The drawing under review shows one solid part. Ordinate dimensions are in mm from its lowest x, y, z. A direction names the side the tool comes from. Give positions to 0.01 mm unless a question says otherwise; leave off trailing zeros. Write each loop counter-clockwise with the first axis right and the second up, starting at its lowest first coordinate (ties: lowest second). Pieces come first, ordered by that corner, then holes. Notation, with made-up numbers: (83, -7.5) -> (117, -7.5) arc R21 cw to (117, 10.5) -> close; hole circle Ø4 at (70, 19). An arc over 180 degrees is marked (long way). Write item = value, one per line.
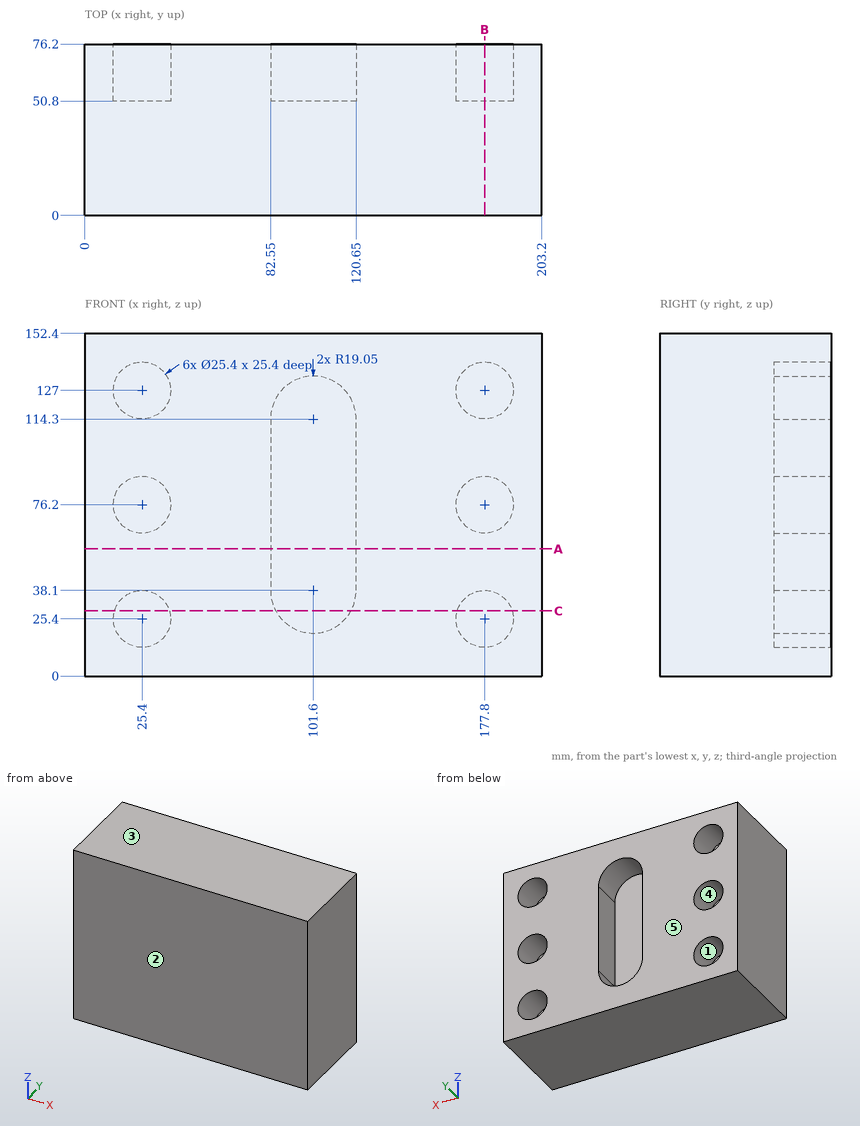
(1) Take a section at C-C (z = 29). Write out the cut boundary in (x, y), plus the area to 3 significant figures.
Answers below:
outline = (0, 0) -> (203.2, 0) -> (203.2, 76.2) -> (189.98, 76.2) -> (189.98, 50.8) -> (165.62, 50.8) -> (165.62, 76.2) -> (118.34, 76.2) -> (118.34, 50.8) -> (84.86, 50.8) -> (84.86, 76.2) -> (37.58, 76.2) -> (37.58, 50.8) -> (13.22, 50.8) -> (13.22, 76.2) -> (0, 76.2) -> close
area = 13,400 mm^2
(2) The part is to be moulded in two halves that separate along Z. For the marked faces 1, 2 and 3, say which applies: released by +Z, released by -Z, zero draft, split by the parting line, or undercut.
Answers below:
face_1 = undercut
face_2 = zero draft
face_3 = released by +Z
(3) To check wall thickness, follow probe 1 along Z at (x, y) = (25.4, 65.75); probe 2 along X at (y, z) = (68, 76); probe 3 along X at (y, z) = (64, 60.5). State the ranges of each line that lie inside material, in increasing order.
Answers below:
probe_1 = 0 to 12.7, 38.1 to 63.5, 88.9 to 114.3, 139.7 to 152.4
probe_2 = 0 to 12.7, 38.1 to 82.55, 120.65 to 165.1, 190.5 to 203.2
probe_3 = 0 to 82.55, 120.65 to 203.2
(4) Take a section at B-B (x = 177.8). Write out the cut boundary in (y, z).
Answers below:
outline = (0, 0) -> (76.2, 0) -> (76.2, 12.7) -> (50.8, 12.7) -> (50.8, 38.1) -> (76.2, 38.1) -> (76.2, 63.5) -> (50.8, 63.5) -> (50.8, 88.9) -> (76.2, 88.9) -> (76.2, 114.3) -> (50.8, 114.3) -> (50.8, 139.7) -> (76.2, 139.7) -> (76.2, 152.4) -> (0, 152.4) -> close
(5) Tool access review of the marked faces 4 and 5: name each direction out of +Z, -Z, +X, -X, +Y, -Y from which nothing blocks a thin tool from reaching the whole face with its end or side.
Answers below:
face_4 = +Y
face_5 = +Z, -Z, +X, -X, +Y
(6) Take a section at A-A (z = 56.5). Write out the cut boundary in (x, y).
Answers below:
outline = (0, 0) -> (203.2, 0) -> (203.2, 76.2) -> (120.65, 76.2) -> (120.65, 50.8) -> (82.55, 50.8) -> (82.55, 76.2) -> (0, 76.2) -> close
(7) For pin 1 (12.5 mm diameter, centred on x = 21, z = 131, fed in from +Y), flat-tipped, find the tip position at first contact; note if it passes through.
Answers below:
pin_1 = 50.8
